CAD build for the part. Positions are in the model's coordinates, mm. A direction names the side the tool comes from. Coordinates: 2 decimals unless noted, no trailing zeros. Loops run counter-clockwise (first coordinate to the right, second up) from the corner with the lowest first, then second, coordinate; pieces in that order, holes last.
1) Which spindle directions (+Z, -Z, +X, -X, +Y, -Y) get a long thin tool onto all of the face, cutting with end or side? Do faces 1 (the flat face through (2, 0, 18)), 2 (the cylindrical face through (5.857, 1.063, 4.38)), 3 (the flat face through (35.8, -0.5, 8.395)). Say none if no direction does.
2) Saw through at C-C, the plane x = 4.5. Give the number of separate pieces and of enclosed holes in the cut face, and give its area (3 significant figures).
3) Wall check: line 1 along Z through (x, y) = (17.5, -0.2); line 2 along X through (y, z) = (1.65, 33.5); line 3 along Z through (x, y) = (35, 1.65). Give the ranges that are in metal, low to high.
4) Two-plate mould, pull along Z, no slides. Class faces 4 (the flat face through (35.7, -0.5, 30.594)), 5 (the flat face through (19.3, -0.5, 0)), 6 (the cylindrical face through (0.8, -0.5, 38.3)), 7 (the flat face through (6, 3.2, 35)): +Z half, -Z half, draft (parallel to the pull), parting line (faces both ways), or undercut.
5) Saw through at B-B, the plane x = 20. Write the cut outline in (y, z), and give its area (3 significant figures).
6) Saw through at D-D, the plane z = 13.5. Write the cut outline in (x, y).
7) Pin check, flat tip, straight feed: pin 1 Ø2.5 at (x, z) = (4.81, 34.18) entering from -Y. Stop position of the tip, or through.
8) Saw through at A-A, the plane y = 0.75. Write the cut outline in (x, z) (1 decimal).
```python
from build123d import *

# Parameters (mm, degrees)
F1_DEPTH = 1.016
F2_R     = 2.8575
F3_DEPTH = 3.2004
F5_D     = 2.2606
F6_R     = 0.635


with BuildPart() as f1:
    # F0 (on Front) → F1 (new body)
    with BuildSketch(Plane.XZ):
        with BuildLine():
            ThreePointArc((0, 2.54), (0.7439487758, 0.7439487758), (2.54, 0))
            Line((2.54, 0), (36.449, 0))
            ThreePointArc((36.449, 0), (38.2450512242, 0.7439487758), (38.989, 2.54))
            Line((38.989, 2.54), (38.989, 8.3947))
            Line((38.989, 8.3947), (32.4780311919, 8.3947))
            ThreePointArc((32.4780311919, 8.3947), (2.413, 19.4945), (32.4780311919, 30.5943))
            Line((32.4780311919, 30.5943), (38.989, 30.5943))
            Line((38.989, 30.5943), (38.989, 36.449))
            ThreePointArc((38.989, 36.449), (38.2450512242, 38.2450512242), (36.449, 38.989))
            Line((36.449, 38.989), (2.54, 38.989))
            ThreePointArc((2.54, 38.989), (0.7439487758, 38.2450512242), (0, 36.449))
            Line((0, 36.449), (0, 2.54))
        make_face()
    extrude(amount=F1_DEPTH)

    # F2 (on face) → F3 (join)
    with BuildSketch(Plane(origin=(0, 0, 0), x_dir=(-1, 0, 0), z_dir=(0, 1, 0))):
        with Locations((-34.1757, 34.1757)):
            Circle(F2_R)
        with Locations((-4.8133, 34.1757)):
            Circle(F2_R)
        with Locations((-4.8133, 4.8133)):
            Circle(F2_R)
        with Locations((-34.1757, 4.8133)):
            Circle(F2_R)
    extrude(amount=F3_DEPTH)

    # F5 (through all)
    with Locations(Plane(origin=(0, 3.2004, 0), x_dir=(-1, 0, 0), z_dir=(0, 1, 0))):
        with Locations((-34.1757, 34.1757), (-4.8133, 4.8133), (-34.1757, 4.8133), (-4.8133, 34.1757)):
            Hole(F5_D / 2)

    # F6
    f6_edges = [f1.edges().sort_by_distance(p)[0] for p in [
        (37.0332, 3.2004, 34.1757),
        (7.6708, 3.2004, 34.1757),
        (7.6708, 3.2004, 4.8133),
        (37.0332, 3.2004, 4.8133),
    ]]
    fillet(f6_edges, radius=F6_R)


solid = f1.part
```
Data:
1. face 1: +Y
1. face 2: +Y, -Y
1. face 3: +X, +Y, -Y
2. separate pieces: 4
2. enclosed holes: 0
2. area: 40.7 mm2
3. line 1: z = 0 to 2.53, 36.46 to 38.99
3. line 2: x = 2.04 to 3.91, 5.72 to 7.59, 31.4 to 33.27, 35.08 to 36.95
3. line 3: z = 2.08 to 4.04, 5.59 to 7.55, 31.44 to 33.4, 34.95 to 36.91
4. face 4: undercut
4. face 5: -Z half
4. face 6: +Z half
4. face 7: draft
5. outline: (-1.02, 0) - (0, 0) - (0, 2.42) - (-1.02, 2.42) - close; (-1.02, 36.57) - (0, 36.57) - (0, 38.99) - (-1.02, 38.99) - close
5. area: 4.92 mm2
6. outline: (0, -1.02) - (3.5, -1.02) - (3.5, 0) - (0, 0) - close
7. pin 1: stops at y = -1.02
8. outline: circle Ø5.7 at (4.8, 4.8); circle Ø5.7 at (4.8, 34.2); circle Ø5.7 at (34.2, 4.8); circle Ø5.7 at (34.2, 34.2); hole circle Ø2.3 at (4.8, 4.8); hole circle Ø2.3 at (4.8, 34.2); hole circle Ø2.3 at (34.2, 4.8); hole circle Ø2.3 at (34.2, 34.2)
